CAD build for the part. Positions are in the model's coordinates, mm. Round coordinates to 2 decimals unless told otherwise and drop trailing zeros. Order: outer loops, then holes, each group sorted by start corner. A loop starts at its lowest first (then second) coordinate and runs counter-clockwise, first axis right, second up. Notation, with made-up numbers: (58.5, 67) - (69.5, 67) arc R6 cw to (69.5, 78) - close; hole circle Ø6 at (75.5, -22.75). An arc over 180 degrees is marked (long way). Use one line per item in the form item = value. Start each with the question number.
from build123d import *

# Parameters (mm, degrees)
BOSS_EXTRUDE1_DEPTH                              = 221
CBORE_FOR_M2_HEX_HEAD_MACHINE_SCREW1_D           = 2.5
CBORE_FOR_M2_HEX_HEAD_MACHINE_SCREW1_CBORE_D     = 4.3
CBORE_FOR_M2_HEX_HEAD_MACHINE_SCREW1_CBORE_DEPTH = 2.5
CHAMFER1_SIZE                                    = 0.3


with BuildPart() as part:
    # Sketch1 → Boss-Extrude1 (new body)
    with BuildSketch(Plane.XY):
        with BuildLine():
            Line((3.5, 4.7), (-3.5, 4.7))
            Line((-3.5, 4.7), (-3.333908129, 4.080136699))
            ThreePointArc((-3.333908129, 4.080136699), (-2.905114055, 3.312564712), (-3.5, 2.665153077))
            Line((-3.5, 2.665153077), (-3.5, 0))
            Line((-3.5, 0), (3.5, 0))
            Line((3.5, 0), (3.5, 2.665153077))
            ThreePointArc((3.5, 2.665153077), (2.905114055, 3.312564712), (3.333908129, 4.080136699))
            Line((3.333908129, 4.080136699), (3.5, 4.7))
        make_face()
    extrude(amount=-BOSS_EXTRUDE1_DEPTH)

    # CBORE for M2 Hex Head Machine Screw1 (through all)
    with Locations(Plane(origin=(0, 4.7, 0), x_dir=(-1, 0, 0), z_dir=(0, 1, 0))):
        with Locations((0, -5.5), (0, -20.5), (0, -35.5), (0, -50.5), (0, -65.5), (0, -80.5), (0, -95.5), (0, -110.5), (0, -125.5), (0, -140.5), (0, -155.5), (0, -170.5), (0, -185.5), (0, -200.5), (0, -215.5)):
            CounterBoreHole(CBORE_FOR_M2_HEX_HEAD_MACHINE_SCREW1_D / 2, CBORE_FOR_M2_HEX_HEAD_MACHINE_SCREW1_CBORE_D / 2, CBORE_FOR_M2_HEX_HEAD_MACHINE_SCREW1_CBORE_DEPTH)

    # Chamfer1
    chamfer1_edges = [part.edges().sort_by_distance(p)[0] for p in [
        (3.5, 0, -110.5),
        (-3.5, 0, -110.5),
    ]]
    chamfer(chamfer1_edges, length=CHAMFER1_SIZE)


solid = part.part
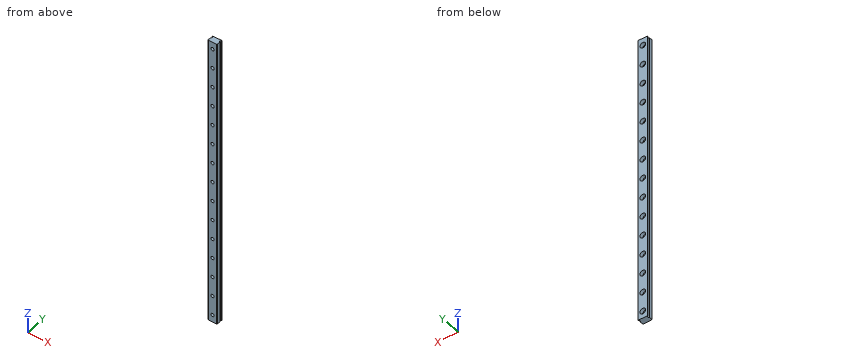
(1) Slice it at A-A (z = -60). Give the cut face in (x, y).
(2) Wall check: line 1 (X direction, y = 2.8, z = -200.5); line 2 (X direction, y = 3.25, z = -215.5); line 3 (X direction, y = 3.95, z = -203). Give the ranges that are in metal, low to high. Write a range as [from, to].
(3) Flat gauge pin, fed straight in: P1, Ø1.3, axis at x = 0.5, z = -6.5, coming from the +Y side. Where does the tip first touch, or does it go through?
(4) Slice it at B-B (x = 0). Give the number of separate pieces and of enclosed holes in the cut face, and give its area (3 significant figures).
Results list:
q1.outline = (-3.5, 0.3) - (-3.2, 0) - (3.2, 0) - (3.5, 0.3) - (3.5, 2.67) arc R0.75 cw to (3.33, 4.08) - (3.5, 4.7) - (-3.5, 4.7) - (-3.33, 4.08) arc R0.75 cw to (-3.5, 2.67) - close
q2.line_1 = [-3.2, -2.15], [2.15, 3.2]
q2.line_2 = [-2.92, -2.15], [2.15, 2.92]
q2.line_3 = [-3.14, 3.14]
q3.P1 = 2.2
q4.separate_pieces = 16
q4.enclosed_holes = 0
q4.area = 795 mm²
